Check sheet for the drawn part. Datum: minimum x, y, z corner. Units: mm. A direction names the side the tool comes from. Give positions to 0.01 mm unless a question says otherwise; leave off trailing zeros. Loops run counter-clockwise (first coordinate to the right, second up) from the corner with the lowest first, then second, coordinate; pieces in that order, holes last. Notation, with made-up numbers: (30.25, 83) - (47.25, 83) arc R30 ccw to (47.25, 111) - close; hole circle Ø10 at (-19, 8.5). An arc over 180 degrees is marked (long way). One line per item, written item: value. Start each with the question number.
1. Scan lines: L1, parallel to X at y = 77.5, z = 3.3; L2, parallel to Z at x = 25, y = 33.5. Record each from-to range of solid material in increasing order. Write a range as [from, to].
2. Sectioned sample at B-B (y = 77.5). Record the cut outline in (x, z).
3. Access from +Z, -Z, +X, -X, +Y, -Y to the whole of each face (thin tool, end or side, straight path). Record for the marked faces 1 and 2.
4. Sectioned sample at D-D (z = 44.5). Record the cut outline in (x, y).
5. Sectioned sample at A-A (x = 30). Record the cut outline in (y, z), plus the area to 3 significant figures.
6. Gauge pin test, flat ends, axial feed: pin 1 (5 mm diameter, centred on x = 34.5, z = 27, fed in from +Y); pin 2 (3 mm diameter, centred on x = 29, z = 46, fed in from -Y); pin 3 (5 mm diameter, centred on x = 45, z = 31.5, fed in from +Y); pin 4 (8 mm diameter, centred on x = 50, y = 88.5, fed in from +Z). Record the tip position at first contact, or that the pin passes through.
7. Sectioned sample at C-C (x = 45). Record the cut outline in (y, z).
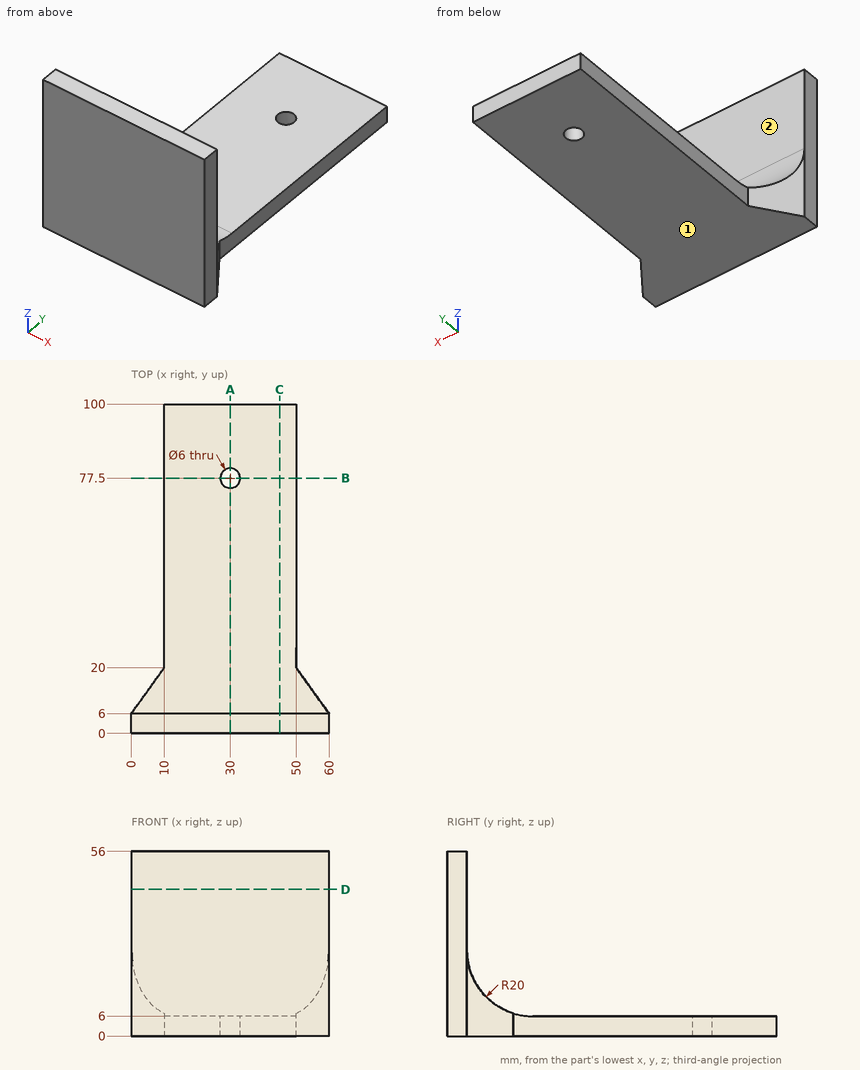
Results are:
1. L1: x = [10, 27], [33, 50]
1. L2: z = [0, 6]
2. outline: (10, 0) - (27, 0) - (27, 6) - (10, 6) - close; (33, 0) - (50, 0) - (50, 6) - (33, 6) - close
3. face 1: -Z, +X, -X, +Y, -Y
3. face 2: +Z, +X, -X, +Y
4. outline: (0, 0) - (60, 0) - (60, 6) - (0, 6) - close
5. outline: (0, 0) - (74.5, 0) - (74.5, 6) - (26, 6) arc R20 cw to (6, 26) - (6, 56) - (0, 56) - close; (80.5, 0) - (100, 0) - (100, 6) - (80.5, 6) - close
5. area: 950 mm^2
6. pin 1: stops at y = 6.06
6. pin 2: stops at y = 0
6. pin 3: stops at y = 6
6. pin 4: stops at z = 6
7. outline: (0, 0) - (100, 0) - (100, 6) - (26, 6) arc R20 cw to (6, 26) - (6, 56) - (0, 56) - close
